Could you check a few things on this model? Use its own coordinates, in mm. Give positions to 0.01 mm unless a question says otherwise; leave off trailing zeros. Loops run counter-clockwise (first coordinate to the right, second up) from the corner with the lowest first, then second, coordinate; pieces in that order, holes last. Notation, with made-up numbers: M 5.25,78 L 47.25,78 A10 cw 47.25,84 Z; hole C 62.5,-5 d4. An arc over 180 degrees is marked long. Use CSV: the item, a comma, the result in double quotes.
```python
from build123d import *

# Parameters (mm, degrees)
SKETCH_W  = 50
SKETCH_H  = 50
SKETCH_R  = 4
PAD_DEPTH = 10


with BuildPart() as part:
    # Sketch → Pad (new body)
    with BuildSketch(Plane.XY):
        Rectangle(SKETCH_W, SKETCH_H)
        with Locations((12.5, 12.5)):
            Circle(SKETCH_R, mode=Mode.SUBTRACT)
        with Locations((-12.5, 12.5)):
            Circle(SKETCH_R, mode=Mode.SUBTRACT)
        with Locations((12.5, -12.5)):
            Circle(SKETCH_R, mode=Mode.SUBTRACT)
        with Locations((-12.5, -12.5)):
            Circle(SKETCH_R, mode=Mode.SUBTRACT)
    pad = extrude(amount=PAD_DEPTH)

    # Mirrored: Pad across face of Pad
    add(pad.mirror(Plane(origin=(25, 0, 5), x_dir=(0, 1, 0), z_dir=(1, 0, 0))))


solid = part.part
```
1. I want a section at D-D, the plane x = 40. List the corners of the cut face in (y, z) for me.
Outcome:
outline,"M -25,0 L -15.62,0 L -15.62,10 L -25,10 Z; M -9.38,0 L 9.38,0 L 9.38,10 L -9.38,10 Z; M 15.62,0 L 25,0 L 25,10 L 15.62,10 Z"
2. I want a section at B-B, the plane x = -12.5. List the corners of the cut face in (y, z) for me.
Outcome:
outline,"M -25,0 L -16.5,0 L -16.5,10 L -25,10 Z; M -8.5,0 L 8.5,0 L 8.5,10 L -8.5,10 Z; M 16.5,0 L 25,0 L 25,10 L 16.5,10 Z"
3. I want a section at C-C, the plane z = 1.25. Give the number of separate pieces and of enclosed holes in the cut face, then the cut area to 3 significant figures.
Outcome:
separate pieces,"1"
enclosed holes,"8"
area,"4,600 mm2"
4. If we mould it in two halves opening along X, with no side actions, what happens to faces 1 (the face through (-25, 0, 5)), 2 (the face through (75, 0, 5)), 3 (the face through (9.3, -14.9, 4.9))? For each: +X half, -X half, draft (parallel to the pull), parting line (faces both ways), or undercut.
Outcome:
face 1,"-X half"
face 2,"+X half"
face 3,"undercut"
5. Please list where these lines run through material, in increasing order: line 1 (Y direction, x = 37.5, z = 6); line 2 (X direction, y = 12, z = 8.25); line 3 (Y direction, x = 10.5, z = 1.75).
Outcome:
line 1,"-25 to -16.5, -8.5 to 8.5, 16.5 to 25"
line 2,"-25 to -16.47, -8.53 to 8.53, 16.47 to 33.53, 41.47 to 58.53, 66.47 to 75"
line 3,"-25 to -15.96, -9.04 to 9.04, 15.96 to 25"
6. I want a section at A-A, the plane y = 12.5. List the corners of the cut face in (x, z) for me, then the cut area to 3 significant figures.
Outcome:
outline,"M -25,0 L -16.5,0 L -16.5,10 L -25,10 Z; M -8.5,0 L 8.5,0 L 8.5,10 L -8.5,10 Z; M 16.5,0 L 33.5,0 L 33.5,10 L 16.5,10 Z; M 41.5,0 L 58.5,0 L 58.5,10 L 41.5,10 Z; M 66.5,0 L 75,0 L 75,10 L 66.5,10 Z"
area,"680 mm2"
